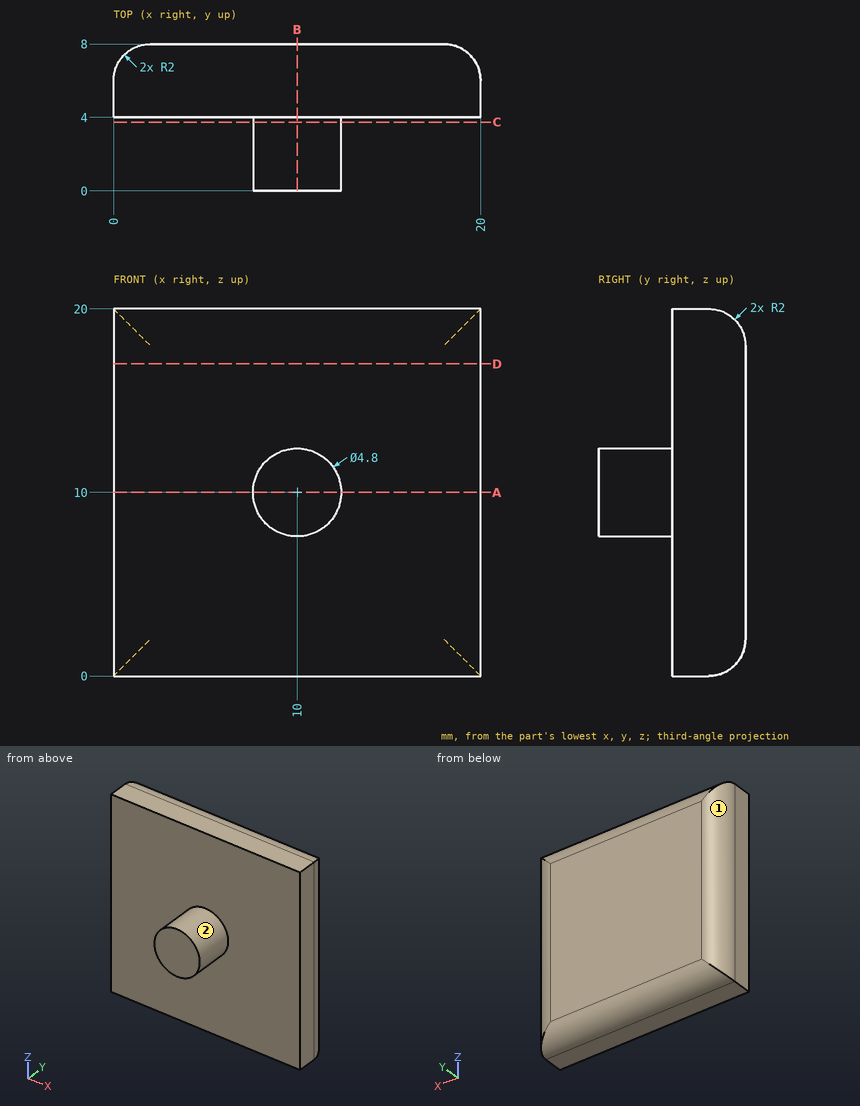
Answer from the drawing. Dimensions are ordinates in mm from the lowest x, y and z of the part. A direction names the side the tool comes from. Give positions to 0.01 mm unless a question says otherwise; leave off trailing zeros. Order: outer loops, then holes, each group sorted by start corner. A loop starts at its lowest first (then second) coordinate and runs counter-clockwise, first axis right, second up. Notation, with made-up numbers: (-9.75, 9) -> (-3.75, 9) arc R12 ccw to (-3.75, 13) -> close; hole circle Ø6 at (72.5, -11). An arc over 180 degrees is marked (long way). One line per item, written item: value. Start each with the question number.
(1) The part is cut by section A-A (z = 10). Determine the outline of the cut face in (x, y), and give its area (3 significant figures).
(2) A tool of negligible diameter and unlimited length cuts with its end or side. For the marked faces 1 and 2, from which of +Z, -Z, +X, -X, +Y, -Y can it reach the whole face along a straight path? Write none if from no direction.
(3) A flat-ended cylindrical pin translates along its axis: P1, Ø1, axis at y = 3, z = 6.5, coming from the +X side. Find the tip coordinate at first contact, or state that the pin passes through.
(4) The part is cut by section D-D (z = 17). Determine the outline of the cut face in (x, y), and give its area (3 significant figures).
(5) The part is cut by section B-B (x = 10). Determine the outline of the cut face in (y, z).
(6) The part is cut by section C-C (y = 3.75). Determine the outline of the cut face in (x, z).
(7) Straight lines are drawn through the part: L1, parallel to Y at x = 12, z = 2.5; L2, parallel to Y at x = 1.5, z = 3; L3, parallel to X at y = 1.25, z = 9.25. For each, find the intervals that lie inside material, in ascending order.
Taken from the geometry:
1. outline: (0, 4) -> (7.6, 4) -> (7.6, 0) -> (12.4, 0) -> (12.4, 4) -> (20, 4) -> (20, 6) arc R2 ccw to (18, 8) -> (2, 8) arc R2 ccw to (0, 6) -> close
1. area: 97.5 mm^2
2. face 1: +Z, -Z, -X, +Y
2. face 2: -Y
3. P1: through
4. outline: (0, 4) -> (20, 4) -> (20, 6) arc R2 ccw to (18, 8) -> (2, 8) arc R2 ccw to (0, 6) -> close
4. area: 78.3 mm^2
5. outline: (0, 7.6) -> (4, 7.6) -> (4, 0) -> (6, 0) arc R2 ccw to (8, 2) -> (8, 18) arc R2 ccw to (6, 20) -> (4, 20) -> (4, 12.4) -> (0, 12.4) -> close
6. outline: circle Ø4.8 at (10, 10)
7. L1: 4 to 8
7. L2: 4 to 7.94
7. L3: 7.72 to 12.28
